For this review, take the finished solid that the model builds, in its own axes (mm). A direction names the side the tool comes from. Coordinates: 2 decimals unless noted, no trailing zeros. Loops run counter-clockwise (first coordinate to the right, second up) from the corner with the lowest first, then second, coordinate; pieces in that order, holes last.
1. Take a section at C-C, the plane z = 33. State the section outline as (x, y) points, then the cut area to 3 significant figures.
2. Machinability: for faces 4 (the face through (19.78, 1.89, -0.85)), 5 (the face through (10, -12.6, 34)), 6 (the face through (19.85, -15.095, 16.121)), which of the approach directions +Z, -Z, +X, -X, +Y, -Y give a long, thin tool a straight path to every point of the face, cutting with its end or side? Answer none if there is none.
3. To check wall thickness, follow probe 1 along Z at (x, y) = (18.5, 1); probe 2 along Z at (x, y) = (15.75, -19.75); probe 3 along Z at (x, y) = (17.5, -1.75). State the ranges of each line that lie inside material, in increasing order.
4. Clearance check with flat-ended pins moving along their axes: P1, Ø2.5, axis at x = 6.5, y = -15.5, coming from the +Z side; P2, Ø6, axis at x = 6.5, y = -5.5, coming from the -Z side; P3, Ø8.5, axis at x = 6, y = 1, coming from the +Z side; P4, Ø6, axis at x = 14.5, y = -13.5, coming from the -Z side. State where each tip first meets the part, or that it passes through.
5. Take a section at D-D, the plane y = -1.5. State the section outline as (x, z) points, then the cut area to 3 significant figures.
6. Take a section at B-B, the plane y = -5.5. State the section outline as (x, z) points.
7. Take a section at A-A, the plane x = 4.5. State the section outline as (y, z) points.
8. Mouldability with a two-part tool opening along Y and no side actions: class faces 1 (the face through (10, 6, 10)), 2 (the face through (10, -17, 22)), 3 (the face through (9.614, -16.705, 6.435)) as pulls with the +Y half, pulls with the -Y half, needs draft (parallel to the pull), parting line crosses it, or undercut.
```python
from build123d import *

# Parameters (mm, degrees)
F0_W     = 10
F0_H     = 25
F1_DEPTH = 20
F2_SIZE  = 0.5
F3_R     = 1.5
F4_R     = 0.5


with BuildPart() as f1:
    # F0 (on Right) → F1 (new body)
    with BuildSketch(Plane.YZ):
        Polygon((3, 0), (0, 0), (3, -1.5), align=None)
        Polygon((3, 19), (3, 0), (3, -1.5), (6, -1.5), (6, 22), (-2.6, 22), (-12.6, 22), (-21.2, 22), (-21.2, -1.5), (-18.2, -1.5), (-18.2, 13.5), (-18.2, 19), (-11.2, 19), align=None)
        Polygon((-18.2, 13.5), (-11.2, 19), (-18.2, 19), align=None)
        with BuildLine():
            ThreePointArc((-18.2, -1.5), (-16.7, 6), (-18.2, 13.5))
            Line((-18.2, 13.5), (-18.2, -1.5))
        make_face()
        with Locations((-7.6, 34.5)):
            Rectangle(F0_W, F0_H)
    extrude(amount=F1_DEPTH)

    # F2
    f2_edges = [f1.edges().sort_by_distance(p)[0] for p in [
        (10, 3, 0),
    ]]
    chamfer(f2_edges, length=F2_SIZE)

    # F3
    f3_edges = [f1.edges().sort_by_distance(p)[0] for p in [
        (10, 3, 19),
        (10, -11.2, 19),
        (10, -18.2, -1.5),
    ]]
    fillet(f3_edges, radius=F3_R)

    # F4
    f4_edges = [f1.edges().sort_by_distance(p)[0] for p in [
        (10, -21.2, 22),
        (10, -21.2, -1.5),
        (0, -21.2, 10.25),
        (20, -21.2, 10.25),
        (20, 3, 9),
        (20, 2.56066, 18.56066),
        (20, 2.75, 0.25),
        (20, -4.590603, 19),
        (20, 1.25, 0),
        (20, -11.171503, 18.917606),
        (20, 1.5, -0.75),
        (20, -14.903969, 16.089739),
        (20, 4.5, -1.5),
        (20, -16.707361, 6.535736),
        (20, 6, 10.25),
        (20, -18.363412, -1.224745),
        (20, 1.7, 22),
        (20, -20.214719, -1.5),
        (20, -2.6, 34.5),
        (20, -7.6, 47),
        (20, -16.9, 22),
        (20, -12.6, 34.5),
        (10, 6, -1.5),
        (10, 6, 22),
        (0, 6, 10.25),
        (10, -2.6, 22),
        (10, -2.6, 47),
        (0, -2.6, 34.5),
        (0, 1.7, 22),
    ]]
    fillet(f4_edges, radius=F4_R)


solid = f1.part
```
Results list:
1. outline: (0, -12.6) - (19.5, -12.6) arc R0.5 ccw to (20, -12.1) - (20, -3.1) arc R0.5 ccw to (19.5, -2.6) - (0.5, -2.6) arc R0.5 ccw to (0, -3.1) - close
1. area: 200 mm2
2. face 4: -Z, +X
2. face 5: +Z, +X, -X, -Y
2. face 6: +X
3. probe 1: z = -0.5 to 0, 19 to 22
3. probe 2: z = -1.5 to 22
3. probe 3: z = 19 to 22
4. P1: stops at z = 22
4. P2: stops at z = 19
4. P3: stops at z = 47
4. P4: stops at z = 14.84
5. outline: (0, 19) - (19.5, 19) arc R0.5 ccw to (20, 19.5) - (20, 21.5) arc R0.5 ccw to (19.5, 22) - (0.5, 22) arc R0.5 ccw to (0, 21.5) - close
5. area: 59.8 mm2
6. outline: (0, 19) - (19.5, 19) arc R0.5 ccw to (20, 19.5) - (20, 46.5) arc R0.5 ccw to (19.5, 47) - (0, 47) - close
7. outline: (-21.2, -1) arc R0.5 ccw to (-20.7, -1.5) - (-19.23, -1.5) arc R1.5 ccw to (-17.82, -0.5) arc R19.5 ccw to (-18.2, 13.5) - (-11.61, 18.68) arc R1.5 cw to (-10.68, 19) - (1.5, 19) arc R1.5 cw to (3, 17.5) - (3, 0.5) - (2.5, 0) - (0, 0) - (3, -1.5) - (5.5, -1.5) arc R0.5 ccw to (6, -1) - (6, 21.5) arc R0.5 ccw to (5.5, 22) - (-2.1, 22) arc R0.5 cw to (-2.6, 22.5) - (-2.6, 46.5) arc R0.5 ccw to (-3.1, 47) - (-12.6, 47) - (-12.6, 22) - (-20.7, 22) arc R0.5 ccw to (-21.2, 21.5) - close
8. face 1: pulls with the +Y half
8. face 2: needs draft
8. face 3: undercut
